from build123d import *

# Parameters (mm, degrees)
BOSS_EXTRU_1_DEPTH                              = 6
CHAMBRAGE_POUR_VIS_T_TE_CYLINDRIQUE_D           = 4.3
CHAMBRAGE_POUR_VIS_T_TE_CYLINDRIQUE_DEPTH       = 14
CHAMBRAGE_POUR_VIS_T_TE_CYLINDRIQUE_CBORE_D     = 8
CHAMBRAGE_POUR_VIS_T_TE_CYLINDRIQUE_CBORE_DEPTH = 4
CHAMBRAGE_POUR_VIS_T_TE_CYLINDRIQUE_TIP         = 1.291850331


with BuildPart() as part:
    # Esquisse2 → Boss.-Extru.1 (new body)
    with BuildSketch(Plane.XY):
        Polygon((-10.964070347, -65), (20.870792038, -377.3), (483.797653512, -377.3), (514.843253, -126.55504147), (514.843253, -17), (125.48114549, -17), (73.48114549, -65), align=None)
        Polygon((11.178308202, -85), (38.93569862, -357.3), (466.12120793, -357.3), (494.843253, -125.321615981), (494.843253, -37), (133.300822179, -37), (81.300822179, -85), align=None, mode=Mode.SUBTRACT)
    extrude(amount=BOSS_EXTRU_1_DEPTH)

    # Chambrage pour vis à tête cylindrique à 6 pans creux (ou vis CHC) M41
    with Locations(Plane.XY.offset(6)):
        with Locations((1.726692055, -145.122614111), (20.068025449, -325.051094707), (130.819543848, -372.8), (260.695946352, -372.8), (410.870792038, -372.8), (494.109580684, -257.391480805), (510.343253, -67.032082447), (364.912339867, -21.5), (194.606610564, -21.5)):
            CounterBoreHole(CHAMBRAGE_POUR_VIS_T_TE_CYLINDRIQUE_D / 2, CHAMBRAGE_POUR_VIS_T_TE_CYLINDRIQUE_CBORE_D / 2, CHAMBRAGE_POUR_VIS_T_TE_CYLINDRIQUE_CBORE_DEPTH, depth=CHAMBRAGE_POUR_VIS_T_TE_CYLINDRIQUE_DEPTH)
            with Locations((0, 0, -(CHAMBRAGE_POUR_VIS_T_TE_CYLINDRIQUE_DEPTH + CHAMBRAGE_POUR_VIS_T_TE_CYLINDRIQUE_TIP / 2))):  # 118° drill point
                Cone(0, CHAMBRAGE_POUR_VIS_T_TE_CYLINDRIQUE_D / 2, CHAMBRAGE_POUR_VIS_T_TE_CYLINDRIQUE_TIP, mode=Mode.SUBTRACT)


solid = part.part
Can you work these out from the model? Positions are in its coordinate system, mm. A direction names the side the tool comes from. Coordinates: 2 decimals unless noted, no trailing zeros. Write each loop counter-clockwise with the first axis right and the second up, starting at its lowest first coordinate (ties: lowest second). Pieces come first, ordered by that corner, then holes. Notation, with made-up numbers: (6, 19.25) - (51, 19.25) arc R34 ccw to (51, 55.25) - close; hole circle Ø5 at (40.5, 71.25). An arc over 180 degrees is marked (long way). Return JSON: item names as keys, results as strings. Group by question number.
Item 1: If we section it at C-C (z = 3): Count the separate pieces of the cut face and the enclosed holes in it, then the cut area to 3 significant figures.
Item 2: Please list where these lines run through material, in increasing order: probe 1 along Y at (x, z) = (128.5, 2.55); probe 2 along Y at (x, z) = (344.5, 3); probe 3 along X at (y, z) = (-372.8, 0.8).
Item 3: Which directions (+Z, -Z, +X, -X, +Y, -Y) give clear straight access to the entire face, cutting with the end or side of a thin tool? Please do faces 4 (the face through (270, -36, 6)), 5 (the face through (480.28, -242.93, 2.96)).
Item 4: I'm going to push flat-ended pins straight in: pin 1 Ø4 at (x, y) = (2.5, -145.5) entering from +Z; pin 2 Ø2.5 at (x, y) = (260.7, -372.8) entering from -Z; pin 3 Ø1 at (y, z) = (-289, 3.5) entering from +X. Where does each tip first touch, or does it pass through?
Item 5: If we section it at B-B (y = -51): Write out the boundary of the cut face in (x, z).
Item 6: If we section it at A-A (x = 172.5): Write out the boundary of the cut face in (y, z), then the cut area to 3 significant figures.
Item 7: We'd pull the mould along Y, two halves only. Please class faces 1 (the face through (270, -36, 0)), 2 (the face through (24.863, -219.244, 2.958)), 3 (the face through (499.1, -253.7, 3)): pulls with the +Y half, pulls with the -Y half, needs draft (parallel to the pull), parting line crosses it, or undercut.
Return value:
{
 "1": {"separate pieces": "1", "enclosed holes": "10", "area": "31,600 mm^2"},
 "2": {"probe 1": "y = -377.3 to -376.06, -369.54 to -357.3, -41.43 to -17", "probe 2": "y = -377.3 to -357.3, -37 to -17", "probe 3": "x = 20.41 to 128.67, 132.97 to 258.55, 262.85 to 408.72, 413.02 to 484.35"},
 "3": {"face 4": "+Z, +X, -X, +Y, -Y", "face 5": "+Z, -Z"},
 "4": {"pin 1": "stops at z = 2", "pin 2": "passes through", "pin 3": "stops at x = 494.79"},
 "5": {"outline": "(88.65, 0) - (118.13, 0) - (118.13, 6) - (88.65, 6) - close; (494.84, 0) - (514.84, 0) - (514.84, 6) - (494.84, 6) - close"},
 "6": {"outline": "(-377.3, 0) - (-357.3, 0) - (-357.3, 6) - (-377.3, 6) - close; (-37, 0) - (-17, 0) - (-17, 6) - (-37, 6) - close", "area": "240 mm^2"},
 "7": {"face 1": "needs draft", "face 2": "undercut", "face 3": "pulls with the -Y half"}
}
